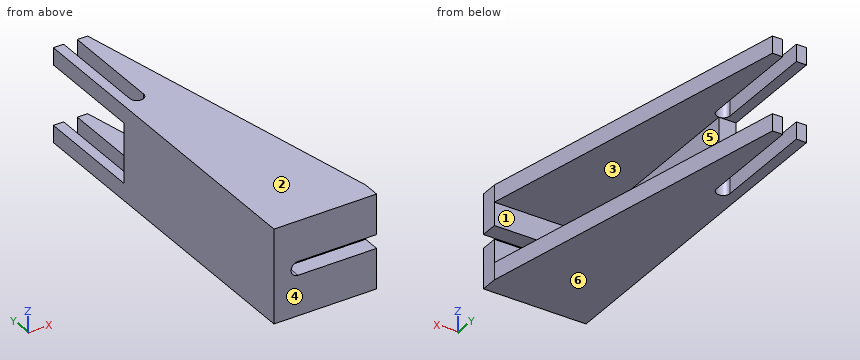
from build123d import *

# Parameters (mm, degrees)
SALIENTE_EXTRUIR1_DEPTH = 55
CORTAR_EXTRUIR1_DEPTH   = 50
CROQUIS4_W              = 35
CROQUIS4_H              = 6.173291601
CORTAR_EXTRUIR2_DEPTH   = 30.5
CORTAR_EXTRUIR3_DEPTH   = 30.5


with BuildPart() as part:
    # Croquis1 → Saliente-Extruir1 (new body)
    with BuildSketch(Plane.XY):
        with BuildLine():
            Line((-28.119282629, 36.435094891), (-28.119282629, -163.564905109))
            Line((-28.119282629, -163.564905109), (31.880717371, -163.564905109))
            Line((31.880717371, -163.564905109), (31.880717371, -153.564905109))
            Line((31.880717371, -153.564905109), (-8.119282629, 36.435094891))
            Line((-8.119282629, 36.435094891), (-14.119282629, 36.435094891))
            Line((-14.119282629, 36.435094891), (-14.119282629, -23.564905109))
            ThreePointArc((-14.119282629, -23.564905109), (-18.119282629, -27.564905109), (-22.119282629, -23.564905109))
            Line((-22.119282629, -23.564905109), (-22.119282629, 36.435094891))
            Line((-22.119282629, 36.435094891), (-28.119282629, 36.435094891))
        make_face()
    extrude(amount=SALIENTE_EXTRUIR1_DEPTH)

    # Croquis2 → Cortar-Extruir1 (cut)
    with BuildSketch(Plane(origin=(31.880717371, 0, 0), x_dir=(0, 0, -1), z_dir=(1, 0, 0))):
        Polygon((-45, -142.180293539), (-45, -153.564905109), (-27.5, -153.564905109), (-10, -153.564905109), (-10, -142.180293539), (-10, 41.509822178), (-45, 41.509822178), align=None)
    extrude(amount=-CORTAR_EXTRUIR1_DEPTH, mode=Mode.SUBTRACT)

    # Croquis4 → Cortar-Extruir2 (cut)
    with BuildSketch(Plane.ZY.offset(28.119282629)):
        with Locations((27.5, 39.521740691)):
            Rectangle(CROQUIS4_W, CROQUIS4_H)
        Polygon((10, -27.564905109), (27.5, -27.564905109), (45, -27.564905109), (45, 36.435094891), (10, 36.435094891), align=None)
    extrude(amount=-CORTAR_EXTRUIR2_DEPTH, mode=Mode.SUBTRACT)

    # Croquis5 → Cortar-Extruir3 (cut)
    with BuildSketch(Plane(origin=(0, -163.564905109, 0), x_dir=(-1, 0, 0), z_dir=(0, -1, 0))):
        with BuildLine():
            Line((-31.880717371, -27.5), (-31.880717371, -31.5))
            Line((-31.880717371, -31.5), (14.119282629, -31.5))
            ThreePointArc((14.119282629, -31.5), (18.119282629, -27.5), (14.119282629, -23.5))
            Line((14.119282629, -23.5), (-31.880717371, -23.5))
            Line((-31.880717371, -23.5), (-31.880717371, -27.5))
        make_face()
    extrude(amount=-CORTAR_EXTRUIR3_DEPTH, mode=Mode.SUBTRACT)


solid = part.part
For this review, take the finished solid that the model builds, in its own axes (mm). Face numbers are marked on the shaded views. A direction names the side the tool comes from. Round coordinates to 2 decimals unless told otherwise and drop trailing zeros. Loops run counter-clockwise (first coordinate to the right, second up) from the corner with the lowest first, then second, coordinate; pieces in that order, holes last. Notation, with made-up numbers: (33.25, 8) - (38.25, 8) arc R17 ccw to (38.25, 17) - close; hole circle Ø1 at (73.5, 76.5). An arc over 180 degrees is marked (long way). One line per item, written item: value. Start each with the question number.
Item 1: Take a section at D-D (x = 1). Give the boundary of the cut face in (y, z).
Item 2: Take a section at C-C (y = -150). Give the boundary of the cut face in (x, z), plus the area to 3 significant figures.
Item 3: For L1, parallel to Z at x = -13.5, y = -23.5; L2, parallel to X at y = -100, z = 15; L3, parallel to Y at x = 19, z = 11.5, list the stretches that pass through material, from the lowest coordinate up.
Item 4: The part is to be moulded in two halves that separate along Z. For the marked faces 3, 4, 5 and 6, say which applies: +Z half, -Z half, draft (parallel to the pull), parting line (faces both ways), or undercut.
Item 5: Clearance check with flat-ended pins moving along their axes: pin 1 Ø12 at (y, z) = (-21, 22.5) entering from +X; pin 2 Ø5 at (y, z) = (11, 48.5) entering from +X; pin 3 Ø5 at (x, z) = (16, 36.5) entering from +Y; pin 4 Ø10 at (y, z) = (-80.5, 18.5) entering from +X. State where each tip first meets the part, or that it passes through.
Item 6: Take a section at A-A (x = 23). Give the boundary of the cut face in (y, z).
Item 7: For the marked faces 1 and 2, list the 3-axis set-ups (+Z, -Z, +X, -X, +Y, -Y) from which the entire face can be reached by the end or side of a thin tool; tool diameter is ignored.
Item 8: Take a section at B-B (z = 17.5). Give the boundary of the cut face in (x, y).
Answer below:
1. outline: (-163.56, 0) - (-6.88, 0) - (-6.88, 10) - (-153.56, 10) - (-153.56, 23.5) - (-163.56, 23.5) - close; (-163.56, 31.5) - (-153.56, 31.5) - (-153.56, 45) - (-6.88, 45) - (-6.88, 55) - (-163.56, 55) - close
2. outline: (-28.12, 0) - (31.13, 0) - (31.13, 10) - (-18.12, 10) - (-18.12, 45) - (31.13, 45) - (31.13, 55) - (-28.12, 55) - close
2. area: 1,530 mm2
3. L1: z = 0 to 10, 45 to 55
3. L2: x = -28.12 to -18.12
3. L3: y = -163.56 to -153.56
4. face 3: undercut
4. face 4: draft
4. face 5: undercut
4. face 6: -Z half
5. pin 1: passes through
5. pin 2: stops at x = -2.24
5. pin 3: stops at y = -153.56
5. pin 4: stops at x = -18.12
6. outline: (-163.56, 0) - (-111.38, 0) - (-111.38, 10) - (-153.56, 10) - (-153.56, 23.5) - (-163.56, 23.5) - close; (-163.56, 31.5) - (-153.56, 31.5) - (-153.56, 45) - (-111.38, 45) - (-111.38, 55) - (-163.56, 55) - close
7. face 1: +X, +Y
7. face 2: +Z, +X, -X, +Y, -Y
8. outline: (-28.12, -163.56) - (31.88, -163.56) - (31.88, -153.56) - (-18.12, -153.56) - (-18.12, -27.56) - (-28.12, -27.56) - close
